Autodesk Inventor part; units mm, degrees
ref_plane "YZ Plane" through (0, 0, 0) normal (1, 0, 0) x (0, 1, 0)
ref_plane "XZ Plane" through (0, 0, 0) normal (0, 1, 0) x (-1, 0, 0)
ref_plane "XY Plane" through (0, 0, 0) normal (0, 0, 1) x (1, 0, 0)
sketch "Sketch1" plane through (0, 0, 0) normal (0, 0, 1) x (1, 0, 0)
  line L0 (0, 96) -> (0, -72)
  line L1 (-18, 0) -> (234, 0)
  line L2 (0, 60) -> (180, 60)
  line L3 (180, 60) -> (180, -60)
  line L4 (180, -60) -> (0, -60)
  line L5 (0, -60) -> (0, 60)
  dimension "d0" = 180
  dimension "d1" = 120
extrude "Extrusion1" add sketch "Sketch1" along normal blind 1
decal "Decal2"
decal "Decal3"
sketch "Sketch5" plane through (0, 0, 1) normal (0, 0, 1) x (1, 0, 0)
  line L0 (0, 60) -> (180, 60)
  line L1 (0, -60) -> (0, 60)
  line L2 (180, -60) -> (0, -60)
  line L3 (0, 38.2522) -> (25.6905, 38.2522)
  line L4 (25.6905, 38.2522) -> (25.6905, 43.1713)
  line L5 (25.6905, 43.1713) -> (19.893, 43.1713)
  line L6 (19.893, 43.1713) -> (19.893, 46.2458)
  line L7 (19.893, 46.2458) -> (21.3863, 48.6175)
  line L8 (21.3863, 48.6175) -> (33.1461, 48.6175)
  line L9 (33.1461, 48.6175) -> (33.1461, 42.5564)
  line L10 (33.1461, 42.5564) -> (35.7923, 42.5564)
  line L11 (35.7923, 42.5564) -> (35.7923, 60)
  line L12 (120.7923, 60) -> (124.7021, 60)
  line L13 (124.7021, 60) -> (124.7021, 40.0365)
  line L14 (124.7021, 40.0365) -> (120.7923, 40.0365)
  line L15 (120.7923, 40.0365) -> (120.7923, 60)
  circle A0 centre (122.7472, 40.0365) radius 1.9549
  line L16 (35.7923, 50.0951) -> (120.7923, 50.0183)
  line L17 (107.7365, 50.0301) -> (109.8537, 50.0301)
  line L18 (109.8537, 50.0301) -> (109.8537, 43.66)
  line L19 (109.8537, 43.66) -> (107.7365, 43.66)
  line L20 (107.7365, 43.66) -> (107.7365, 50.0301)
  circle A1 centre (108.7951, 43.66) radius 1.0586
  dimension "d14" = 85
extrude "Extrusion2" cut sketch "Sketch5" against normal through all
sketch "Sketch6" plane through (0, 0, 1) normal (0, 0, 1) x (1, 0, 0)
  line L0 (124.7021, 60) -> (124.7021, 40.0365)
  line L1 (0, -60) -> (0, 38.2522)
  line L2 (180, -60) -> (0, -60)
  line L3 (180, 60) -> (180, -60)
  line L4 (124.7021, 60) -> (180, 60)
  line L5 (124.7021, 46.8108) -> (132.4781, 46.8108)
  line L6 (132.4781, 46.8108) -> (132.4781, 38.2477)
  line L7 (168, -50) -> (0, -50)
  line L8 (-18, 0) -> (234, 0)
  line L9 (168, 43) -> (168, -50)
  line L10 (132.4781, 38.2477) -> (150.9588, 38.2477)
  line L11 (150.9588, 38.2477) -> (150.9588, 43)
  line L12 (150.9588, 43) -> (168, 43)
  dimension "d16" = 93
  dimension "d17" = 10
  dimension "d18" = 168
extrude "Extrusion3" cut sketch "Sketch6" against normal through all contours L4 L3 L8 L9 L12 L11 L10 L6 L5 L0 | L3 L2 L1 L7 L9 L8
sketch "Sketch3" plane through (0, 0, 1) normal (0, 0, 1) x (1, 0, 0)
  line L0 (0, 50.1511) -> (168, 50.1511) construction
  line L1 (168, 50.1511) -> (168, -50.153) construction
  line L2 (168, -50.153) -> (0, -50.153) construction
  line L3 (0, -50.153) -> (0, 50.1511) construction
  point P0 (0, 0)
  point P1 (0, 0)
sketch "Sketch4" plane through (0, 0, 0) normal (0, 0, -1) x (-1, 0, 0)
  line L0 (0, -60) -> (0, 60)
  line L1 (-165.5, 50.5194) -> (0, 50.5194) construction
  line L2 (0, 50.5194) -> (0, -50.5196) construction
  line L3 (0, -50.5196) -> (-165.5, -50.5196) construction
  line L4 (-165.5, -50.5196) -> (-165.5, 50.5194) construction
  point P0 (0, 0)
  point P1 (0, 0)
  point P2 (0, -50.5196)
properties part number "config - graphic card"
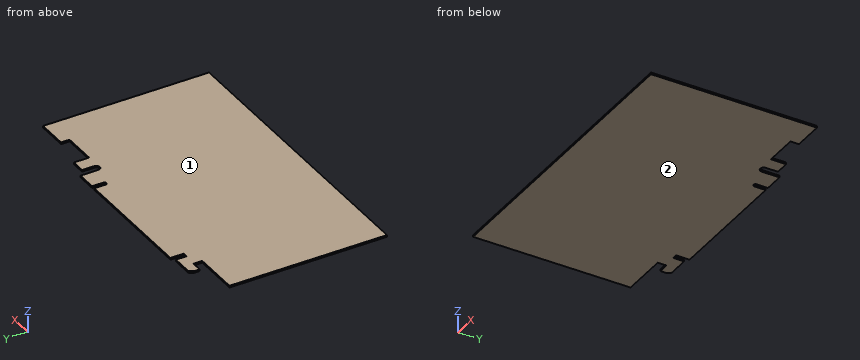
For this review, take the finished solid that the model builds, in its own axes (mm). Face numbers are marked on the shaded views. Round coordinates to 2 decimals unless told otherwise and drop trailing zeros. Loops run counter-clockwise (first coordinate to the right, second up) from the corner with the lowest first, then second, coordinate; pieces in that order, holes last. Notation, with made-up numbers: (75, -31.75) - (118, -31.75) arc R22 ccw to (118, -23.75) - close; hole circle Ø9 at (85, 19). An arc over 180 degrees is marked (long way). One line per question, with ' | ' between items.
Q1. For pin 1 (5 mm diameter, centred on x = 54.5, y = -7.5, fed in from -Z); pin 2 (0.5 mm diameter, centred on x = 34.5, z = 0.5, fed in from +Y); pin 3 (0.5 mm diameter, centred on x = 27, z = 0.5, fed in from +Y), all flat-tipped, find the tip position at first contact; note any pin that passes through.
Taken from the geometry:
pin 1: stops at z = 0 | pin 2: stops at y = 42.56 | pin 3: stops at y = 48.62
Q2. The part is to be moulded in two halves that separate along Z. For the marked faces 1 and 2, say which applies: released by +Z, released by -Z, zero draft, split by the parting line, or undercut.
Taken from the geometry:
face 1: released by +Z | face 2: released by -Z
Q3. Take a section at A-A (z = 0.65). Give the boundary of the cut face in (x, y), and give its area (3 significant figures).
Taken from the geometry:
outline: (0, -50) - (168, -50) - (168, 43) - (150.96, 43) - (150.96, 38.25) - (132.48, 38.25) - (132.48, 46.81) - (124.7, 46.81) - (124.7, 40.04) arc R1.95 cw to (120.79, 40.04) - (120.79, 50.02) - (109.85, 50.03) - (109.85, 43.66) arc R1.06 cw to (107.74, 43.66) - (107.74, 50.03) - (35.79, 50.1) - (35.79, 42.56) - (33.15, 42.56) - (33.15, 48.62) - (21.39, 48.62) - (19.89, 46.25) - (19.89, 43.17) - (25.69, 43.17) - (25.69, 38.25) - (0, 38.25) - close | area: 16,100 mm²
Q4. For line 1 along Y through (x, z) = (94.5, 0.25); line 2 along Y through (x, z) = (7, 0.85), list the stretches that pass through material, from the lowest coordinate up. Write a range as [from, to].
Taken from the geometry:
line 1: y = [-50, 50.04] | line 2: y = [-50, 38.25]
